Part model, mm, in its own coordinate system. Face numbers are marked on the shaded views. A direction names the side the tool comes from. Round coordinates to 2 decimals unless told otherwise and drop trailing zeros. Loops run counter-clockwise (first coordinate to the right, second up) from the corner with the lowest first, then second, coordinate; pieces in that order, holes last.
from build123d import *

# Parameters (mm, degrees)
BOSS_EXTRUDE1_DEPTH        = 1.7
SKETCH2_W                  = 26
SKETCH2_H                  = 1.7
BOSS_EXTRUDE2_DEPTH        = 29.2
F_10_0_10_DIAMETER_HOLE1_D = 10
F_3_0_3_DIAMETER_HOLE1_D   = 3
F_10_0_10_DIAMETER_HOLE2_D = 10
F_3_0_3_DIAMETER_HOLE2_D   = 3
FILLET1_R                  = 2.5


with BuildPart() as part:
    # Sketch1 → Boss-Extrude1 (new body)
    with BuildSketch(Plane(origin=(0, -13.75, 0), x_dir=(1, 0, 0), z_dir=(0, 1, 0))):
        with BuildLine():
            Line((13.000000223, -17.8), (13.000000223, 0))
            Line((13.000000223, 0), (-13, 0))
            Line((-13, 0), (-13, -17.8))
            ThreePointArc((-13, -17.8), (-9.198386918, -27.027675803), (1.11e-07, -30.899618316))
            ThreePointArc((1.11e-07, -30.899618316), (9.19838714, -27.027675803), (13.000000223, -17.8))
        make_face()
    extrude(amount=-BOSS_EXTRUDE1_DEPTH)

    # Sketch2 → Boss-Extrude2 (add)
    with BuildSketch(Plane(origin=(0, -13.75, 0), x_dir=(-1, 0, 0), z_dir=(0, 1, 0))):
        with Locations((0, 0.85)):
            Rectangle(SKETCH2_W, SKETCH2_H)
    extrude(amount=BOSS_EXTRUDE2_DEPTH)

    # Ø10.0 (10) Diameter Hole1 (through all)
    with Locations(Plane(origin=(0, -13.75, 0), x_dir=(1, 0, 0), z_dir=(0, 1, 0))):
        with Locations((-0.099999806, -19.5)):
            Hole(F_10_0_10_DIAMETER_HOLE1_D / 2)

    # Ø3.0 (3) Diameter Hole1 (through all)
    with Locations(Plane(origin=(0, -13.75, 0), x_dir=(1, 0, 0), z_dir=(0, 1, 0))):
        with Locations((8.5, -19.5), (-8.5, -19.5)):
            Hole(F_3_0_3_DIAMETER_HOLE1_D / 2)

    # Ø10.0 (10) Diameter Hole2 (through all)
    with Locations(Plane.XY.offset(1.7)):
        with Locations((0.1, 0.05)):
            Hole(F_10_0_10_DIAMETER_HOLE2_D / 2)

    # Ø3.0 (3) Diameter Hole2 (through all)
    with Locations(Plane.XY.offset(1.7)):
        with Locations((-7.8, 6.95), (8, -6.95), (-7.8, -6.95), (8, 6.95)):
            Hole(F_3_0_3_DIAMETER_HOLE2_D / 2)

    # Fillet1
    fillet1_edges = [part.edges().sort_by_distance(p)[0] for p in [
        (1.11e-07, -15.45, 0),
        (0, -13.75, 1.7),
    ]]
    fillet(fillet1_edges, radius=FILLET1_R)


solid = part.part
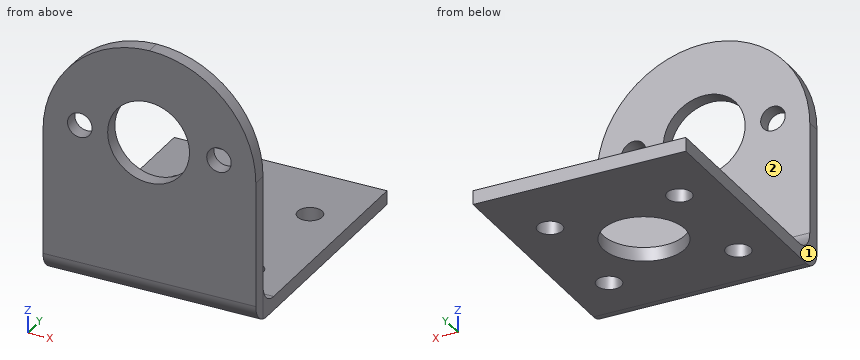
1) Slice it at A-A, the plane x = -1. Give the cut face in (y, z), then the cut area to 3 significant figures.
Values:
outline: (-15.45, 2.5) arc R2.5 ccw to (-12.95, 0) - (-4.83, 0) - (-4.83, 1.7) - (-11.25, 1.7) arc R2.5 cw to (-13.75, 4.2) - (-13.75, 14.58) - (-15.45, 14.58) - close; (-15.45, 24.42) - (-13.75, 24.42) - (-13.75, 30.85) - (-15.45, 30.85) - close; (4.93, 0) - (15.45, 0) - (15.45, 1.7) - (4.93, 1.7) - close
area: 68.8 mm2
2) Tool access for the marked faces 1 and 2: list every direction of +Z, -Z, +X, -X, +Y, -Y with a clear straight run to the whole face (end or side of a thin tool).
Values:
face 1: +Z, -Z, -X, +Y, -Y
face 2: +Z, +X, -X, +Y
3) Slice it at D-D, the plane x = -8.25. Give the cut face in (y, z).
Values:
outline: (-15.45, 2.5) arc R2.5 ccw to (-12.95, 0) - (-8.38, 0) - (-8.38, 1.7) - (-11.25, 1.7) arc R2.5 cw to (-13.75, 4.2) - (-13.75, 18.02) - (-15.45, 18.02) - close; (-15.45, 20.98) - (-13.75, 20.98) - (-13.75, 27.89) - (-15.45, 27.89) - close; (-5.52, 0) - (5.52, 0) - (5.52, 1.7) - (-5.52, 1.7) - close; (8.38, 0) - (15.45, 0) - (15.45, 1.7) - (8.38, 1.7) - close
4) Slice it at C-C, the plane z = 20. Give the cut face in (x, y), then the cut area to 3 significant figures.
Values:
outline: (-12.81, -15.45) - (-9.91, -15.45) - (-9.91, -13.75) - (-12.81, -13.75) - close; (-7.09, -15.45) - (-5.07, -15.45) - (-5.07, -13.75) - (-7.09, -13.75) - close; (4.87, -15.45) - (7.09, -15.45) - (7.09, -13.75) - (4.87, -13.75) - close; (9.91, -15.45) - (12.81, -15.45) - (12.81, -13.75) - (9.91, -13.75) - close
area: 17.0 mm2
5) Wall check: line 1 along Y through (x, z) = (8, 0.85); line 2 along X through (y, z) = (-15, 19); line 3 along Y through (x, z) = (-7.8, 1.1). Give the ranges that are in metal, low to high.
Values:
line 1: y = -14.83 to -8.45, -5.45 to 5.45, 8.45 to 15.45
line 2: x = -12.94 to -9.91, -7.09 to -5.07, 4.87 to 7.09, 9.91 to 12.94
line 3: y = -15.02 to -8.45, -5.45 to 5.45, 8.45 to 15.45
6) Drop flat-ended pins along their axis: pin 1 Ø1.5 at (x, y) = (6.5, -9) entering from +Z; pin 2 Ø1 at (x, y) = (3, -12) entering from +Z. Give the stop position or say it passes through.
Values:
pin 1: stops at z = 1.7
pin 2: stops at z = 2.03
7) Slice it at B-B, the plane y = -6.95. Give the cut face in (x, z), then the cut area to 3 significant figures.
Values:
outline: (-13, 0) - (-9.3, 0) - (-9.3, 1.7) - (-13, 1.7) - close; (-6.3, 0) - (6.5, 0) - (6.5, 1.7) - (-6.3, 1.7) - close; (9.5, 0) - (13, 0) - (13, 1.7) - (9.5, 1.7) - close
area: 34.0 mm2
